```python
from build123d import *

# Parameters (mm, degrees)
SKETCH1_R           = 2.032
SKETCH1_R_2         = 2.286
SKETCH1_R_3         = 2.0955
SKETCH1_W           = 4.445
SKETCH1_H           = 4.445
BOSS_EXTRUDE1_DEPTH = 3.175
FILLET1_R           = 4.7625


with BuildPart() as part:
    # Sketch1 → Boss-Extrude1 (new body)
    with BuildSketch(Plane.XY):
        with BuildLine():
            Line((-9.525, -30.48), (-9.525, 20.32))
            Line((-9.525, 20.32), (9.525, 20.32))
            ThreePointArc((9.525, 20.32), (15.760681597, 9.08548638), (26.69688421, 2.340303383))
            ThreePointArc((26.69688421, 2.340303383), (30.065673036, -2.173245584), (26.774154282, -6.743449816))
            ThreePointArc((26.774154282, -6.743449816), (14.292700247, -15.808964436), (9.525, -30.48))
            Line((9.525, -30.48), (-9.525, -30.48))
        make_face()
        with Locations((25.303345332, -2.213755866)):
            Circle(SKETCH1_R, mode=Mode.SUBTRACT)
        with Locations((0, 12.7)):
            Circle(SKETCH1_R_2, mode=Mode.SUBTRACT)
        Circle(SKETCH1_R_3, mode=Mode.SUBTRACT)
        with Locations((0, -25.4)):
            Rectangle(SKETCH1_W, SKETCH1_H, mode=Mode.SUBTRACT)
        with Locations((0, -12.7)):
            Rectangle(SKETCH1_W, SKETCH1_H, mode=Mode.SUBTRACT)
    extrude(amount=BOSS_EXTRUDE1_DEPTH)

    # Fillet1
    fillet1_edges = [part.edges().sort_by_distance(p)[0] for p in [
        (-9.525, -30.48, 1.5875),
        (-9.525, 20.32, 1.5875),
        (9.525, 20.32, 1.5875),
        (9.525, -30.48, 1.5875),
    ]]
    fillet(fillet1_edges, radius=FILLET1_R)


solid = part.part
```
Part model, mm, in its own coordinate system. A direction names the side the tool comes from. Round coordinates to 2 decimals unless told otherwise and drop trailing zeros. Write each loop counter-clockwise with the first axis right and the second up, starting at its lowest first coordinate (ties: lowest second). Pieces come first, ordered by that corner, then holes. Notation, with made-up numbers: (-15.5, 45) -> (8.5, 45) arc R20 cw to (8.5, 60) -> close; hole circle Ø8 at (-19.75, -38.5). An arc over 180 degrees is marked (long way). Return JSON: item names as keys, results as strings. Group by question number.
Q1. Which spindle directions (+Z, -Z, +X, -X, +Y, -Y) get a long thin tool onto all of the face, cutting with end or side? Do faces 4 (the flat face through (2.222, -13, 2)), 5 (the cylindrical face through (16.774, 8.083, 1.565)). Say none if no direction does.
Q2. Saw through at D-D on y = 12.7. Write the cut outline in (x, z) (3 decimals).
Q3. Probe L1, parallel to Y at x = 0, z = 1.1; L2, parallel to X at y = -11, z = 2.3 (1 decimal); L3, parallel to X at y = 13.5, z = 2.8 (3 decimals). List the from-to ranges inside material, lowest first. Write a range as [from, to].
Q4. Saw through at C-C on z = 1.2. Write the cut outline in (x, y) (1 decimal).
Q5. Saw through at B-B on y = -3.5. Write the cut outline in (x, z) (3 decimals), plus the area to 3 significant figures.
Q6. Saw through at A-A on x = 0. Write the cut outline in (y, z) (1 decimal), plus the area to 3 significant figures.
Q7. Mould opens along Y. For faces 1 (the cylindrical face through (15.66, -14.09, 1.57)), 2 (the cylindrical face through (2, 0.63, 1.57)), 3 (the flat face through (6, -5, 0)) say: pulls with the +Y half, pulls with the -Y half, needs draft (parallel to the pull), parting line crosses it, or undercut.
Q8. Pin check, flat tips, straight feed: pin 1 (3.5 mm diameter, centred on x = 0, y = 0, fed in from -Z); pin 2 (1.6 mm diameter, centred on y = -12.5, z = 1, fed in from +X); pin 3 (1.6 mm diameter, centred on y = -26, z = 2.5, fed in from +X). Stop position of each tip, or through.
Answer:
{
 "1": {"face 4": "+Z, -Z", "face 5": "+Z, -Z, +X, +Y"},
 "2": {"outline": "(-9.525, 0) -> (-2.286, 0) -> (-2.286, 3.175) -> (-9.525, 3.175) -> close; (2.286, 0) -> (12.889, 0) -> (12.889, 3.175) -> (2.286, 3.175) -> close"},
 "3": {"L1": "[-30.48, -27.62], [-23.18, -14.92], [-10.48, -2.1], [2.1, 10.41], [14.99, 20.32]", "L2": "[-9.5, -2.2], [2.2, 18.9]", "L3": "[-9.525, -2.141], [2.141, 12.385]"},
 "4": {"outline": "(-9.5, -25.7) arc R4.8 ccw to (-4.8, -30.5) -> (5.1, -30.5) arc R4.8 ccw to (9.8, -26.5) arc R25 cw to (26.8, -6.7) arc R4.8 ccw to (26.7, 2.3) arc R25.4 cw to (10.5, 17.3) arc R4.8 ccw to (6.1, 20.3) -> (-4.8, 20.3) arc R4.8 ccw to (-9.5, 15.6) -> close; hole circle Ø4.6 at (0, 12.7); hole (-2.2, -27.6) -> (2.2, -27.6) -> (2.2, -23.2) -> (-2.2, -23.2) -> close; hole (-2.2, -14.9) -> (2.2, -14.9) -> (2.2, -10.5) -> (-2.2, -10.5) -> close; hole circle Ø4.2 at (0, 0); hole circle Ø4.1 at (25.3, -2.2)"},
 "5": {"outline": "(-9.525, 0) -> (23.73, 0) -> (23.73, 3.175) -> (-9.525, 3.175) -> close; (26.876, 0) -> (29.889, 0) -> (29.889, 3.175) -> (26.876, 3.175) -> close", "area": "115 mm2"},
 "6": {"outline": "(-30.5, 0) -> (-27.6, 0) -> (-27.6, 3.2) -> (-30.5, 3.2) -> close; (-23.2, 0) -> (-14.9, 0) -> (-14.9, 3.2) -> (-23.2, 3.2) -> close; (-10.5, 0) -> (-2.1, 0) -> (-2.1, 3.2) -> (-10.5, 3.2) -> close; (2.1, 0) -> (10.4, 0) -> (10.4, 3.2) -> (2.1, 3.2) -> close; (15, 0) -> (20.3, 0) -> (20.3, 3.2) -> (15, 3.2) -> close", "area": "105 mm2"},
 "7": {"face 1": "pulls with the -Y half", "face 2": "undercut", "face 3": "needs draft"},
 "8": {"pin 1": "through", "pin 2": "x = 18.05", "pin 3": "x = 10.09"}
}
